The listing builds one solid part. Answer for the finished solid, in the listing's coordinates (mm). A direction names the side the tool comes from. Coordinates: 2 decimals unless noted, no trailing zeros. Order: outer loops, then holes, each group sorted by start corner. A loop starts at its lowest first (then second) coordinate and runs counter-clockwise, first axis right, second up. Notation, with made-up numbers: M -26.5,-27 L -16.5,-27 A20 cw -16.5,-19 Z; hole C 44.5,-4.75 d3. An arc over 180 degrees is marked long. One line per item, written item: value. Start each with the question number.
Q1. For faces 4 (the flat face through (-15, 4.5, -2)), 5 (the cylindrical face through (-18.928, 7.288, -0.729)), determine the directions among +Z, -Z, +X, -X, +Y, -Y from which every point of the face is accessible in a straight line to the end or side of a thin tool.
Q2. This flat-tipped pin is pushed along its axis until it touches: pin 1 Ø3.5 at (x, z) = (14.5, -0.5) entering from -Y. Where does it stop, or does it pass through?
Q3. Straight lines are drawn through the part: line 1 along Z through (x, y) = (-17, 0.5); line 2 along Z through (x, y) = (-14.5, 5.5); line 3 along X through (y, z) = (1.25, 12). For each, find the intervals that lie inside material, in ascending order. Write a range as [from, to].
Q4. Determine the mould class of faces 1 (the cylindrical face through (-2.153, 7.212, 11.444)), 2 (the flat face through (14, 5, 24.361)), 3 (the flat face through (-31.88, 5, 10)) for opening direction Z: pulls with the +Z half, pulls with the -Z half, needs draft (parallel to the pull), parting line crosses it, or undercut.
Q5. The part is cut by section A-A on x = 28. Give the vertices of the cut face in (y, z).
Q6. The part is cut by section B-B on y = 5.75. Give the number of separate pieces and of enclosed holes in the cut face, then the cut area to 3 significant figures.
Autodesk Inventor part; units mm, degrees
ref_plane "YZ Plane" through (0, 0, 0) normal (1, 0, 0) x (0, 1, 0)
ref_plane "XZ Plane" through (0, 0, 0) normal (0, 1, 0) x (-1, 0, 0)
ref_plane "XY Plane" through (0, 0, 0) normal (0, 0, 1) x (1, 0, 0)
sketch "Sketch1" plane through (0, 0, 0) normal (0, 1, 0) x (-1, 0, 0)
  line L0 (31.8795, -5.6386) -> (-58.1205, -5.6386)
  line L1 (-58.1205, -5.6386) -> (-58.1205, 24.3614)
  line L2 (-58.1205, 24.3614) -> (31.8795, 24.3614)
  line L3 (31.8795, 24.3614) -> (31.8795, -5.6386)
  point P0 (0, 0)
  dimension "d0" = 90
  dimension "d5" = 30
extrude "Extrusion1" add sketch "Sketch1" along normal blind 10
sketch "Sketch2" plane through (0, 10, 0) normal (0, 1, 0) x (1, 0, 0)
  line L0 (58.1205, 5.6386) -> (-31.8795, 5.6386)
  line L1 (-31.8795, 5.6386) -> (-31.8795, -24.3614)
  circle A0 centre (-16.8795, 0.6386) radius 2.05
  circle A1 centre (13.1205, 0.6386) radius 2.05
  circle A2 centre (43.1205, 0.6386) radius 2.05
  point P0 (0, 0)
  dimension "d8" = 4.1
  dimension "d10" = 4.1
  dimension "d11" = 4.1
  dimension "d12" = 5
  dimension "d13" = 5
  dimension "d14" = 5
  dimension "d15" = 15
  dimension "d16" = 30
  dimension "d17" = 30
extrude "Extrusion2" cut sketch "Sketch2" against normal blind 10
sketch "Sketch4" plane through (0, 0, 0) normal (0, -1, 0) x (1, 0, 0)
  circle A0 centre (13.1205, -0.6386) radius 2.05
  circle A1 centre (-16.8795, -0.6386) radius 2.05
  circle A2 centre (43.1205, -0.6386) radius 2.05
  circle A3 centre (-16.8795, -0.6386) radius 3.5
  circle A4 centre (13.1205, -0.6386) radius 3.5
  circle A5 centre (43.1205, -0.6386) radius 3.5
  point P0 (0, 0)
  dimension "d26" = 7
  dimension "d28" = 7
  dimension "d29" = 7
extrude "Extrusion4" cut sketch "Sketch4" against normal blind 4.5
sketch "Sketch5" plane through (0, 0, 0) normal (0, -1, 0) x (1, 0, 0)
  line L0 (58.1205, -5.6386) -> (58.1205, 24.3614)
  line L1 (58.1205, 24.3614) -> (-31.8795, 24.3614)
  line L2 (-31.8795, 24.3614) -> (-31.8795, -5.6386)
  circle A0 centre (-1.8795, 9.3614) radius 2.1
  circle A1 centre (28.1205, 9.3614) radius 2.1
  point P0 (0, 0)
  dimension "d32" = 4.2
  dimension "d34" = 4.2
  dimension "d35" = 30
  dimension "d36" = 30
  dimension "d37" = 15
  dimension "d38" = 15
extrude "Extrusion5" cut sketch "Sketch5" against normal blind 10
sketch "Sketch6" plane through (0, 0, 0) normal (0, -1, 0) x (1, 0, 0)
  circle A0 centre (-1.8795, 9.3614) radius 2.1
  circle A1 centre (28.1205, 9.3614) radius 2.1
  circle A2 centre (-1.8795, 9.3614) radius 3.5
  circle A3 centre (28.1205, 9.3614) radius 3.5
  point P0 (0, 0)
  dimension "d41" = 7
  dimension "d43" = 7
extrude "Extrusion6" cut sketch "Sketch6" against normal blind 4.5
sketch "Sketch7" plane through (0, 10, 0) normal (0, 1, 0) x (1, 0, 0)
  line L0 (-31.8795, -24.3614) -> (58.1205, -24.3614)
  line L1 (58.1205, -24.3614) -> (58.1205, 5.6386)
  circle A0 centre (45.6205, -9.8614) radius 1.25
  circle A1 centre (15.6205, -9.8614) radius 1.25
  circle A2 centre (-14.3795, -9.8614) radius 1.25
  point P0 (0, 0)
  dimension "d46" = 2.5
  dimension "d48" = 2.5
  dimension "d49" = 2.5
  dimension "d50" = 12.5
  dimension "d51" = 14.5
  dimension "d52" = 30
  dimension "d53" = 30
  dimension "d54" = 14.5
  dimension "d55" = 14.5
extrude "Extrusion7" cut sketch "Sketch7" against normal blind 20
equation "\"d10\" = d8"
equation "\"d11\" = d8"
equation "\"d13\" = d12"
equation "\"d14\" = d12"
equation "\"d28\" = d26"
equation "\"d29\" = d26"
properties part number "AgarMouldBottomV3"
Output:
1. face 4: -Y
1. face 5: +Y, -Y
2. pin 1: stops at y = 4.5
3. line 1: z = [-5.64, -4.14], [2.86, 24.36]
3. line 2: z = [-5.64, 8.62], [11.11, 24.36]
3. line 3: x = [-31.88, -4.18], [0.42, 25.82], [30.42, 58.12]
4. face 1: undercut
4. face 2: pulls with the +Z half
4. face 3: needs draft
5. outline: M 0,-5.64 L 10,-5.64 L 10,7.26 L 4.5,7.26 L 4.5,5.86 L 0,5.86 Z; M 0,12.86 L 4.5,12.86 L 4.5,11.46 L 10,11.46 L 10,24.36 L 0,24.36 Z
6. separate pieces: 1
6. enclosed holes: 8
6. area: 2,620 mm^2
